Model file for the job. Use its own axes, mm. A direction names the side the tool comes from. Give positions to 0.01 mm unless a question says otherwise; leave off trailing zeros. Loops run counter-clockwise (first coordinate to the right, second up) from the corner with the lowest first, then second, coordinate; pieces in that order, holes last. Notation, with made-up numbers: (5, -39.75) -> (61, -39.75) arc R22 cw to (61, -19.75) -> close; hole circle Ø2 at (62.25, 73.25). An arc over 180 degrees is marked (long way). Use CSV: the item, a comma, the result in double quotes. Start each with the question number.
(1) Cut at C-C on y = 44. Write the cut outline in (x, z), then the cut area to 3 significant figures.
(2) Flat gauge pin, fed straight in: pin 1 (7.5 mm diameter, centred on x = 19.5, y = -65, fed in from +Z). Where does the tip first touch, or does it go through?
(3) Cut at A-A on y = -65. Write the cut outline in (x, z), then the cut area to 3 significant figures.
(4) 3-axis set-ups, long thin cutter, end or side, ignore diameter. For faces 4 (the flat face through (-21.4, -65.2, 3)), 5 (the flat face through (-19, 60, 1)), 6 (the flat face through (25.2, 0.3, 10)): which of +Z, -Z, +X, -X, +Y, -Y reach the whole face in a straight line?
(5) Drill centre lines: probe 1 along Y at (x, z) = (-19, 1.7); probe 2 along X at (y, z) = (65, 1.85); probe 3 along X at (y, z) = (-62.5, 3.75). Where is each one in solid material? Low to high.
(6) Cut at B-B on x = 4. Write the cut outline in (y, z).
(7) Cut at D-D on z = 6.25. Write the cut outline in (x, y), then the cut area to 3 significant figures.
(8) Pull direction X, two halves, no side cores. Call faces 1 (the flat face through (0, 70, 5)), 2 (the flat face through (26, 6, 0)), 3 (the flat face through (-27, -1, 4)): pulls with the +X half, pulls with the -X half, needs draft (parallel to the pull), parting line crosses it, or undercut.
Solid Edge part; units mm, degrees
sketch "Sketch1" plane through (0, 0, 0) normal (0, 0, 1) x (1, 0, 0)
  line L0 (27, -73) -> (-27, -73)
  line L1 (-27, -73) -> (-27, 73)
  line L2 (-27, 73) -> (27, 73)
  line L3 (27, 73) -> (27, -73)
  dimension "D1" = 27
  dimension "D2" = 27
extrude "Protrusion1" add sketch "Sketch1" along normal blind 10
sketch "Sketch2" plane through (0, 0, 10) normal (0, 0, 1) x (1, 0, 0)
  line L0 (24, -70) -> (-24, -70)
  line L1 (-24, -70) -> (-24, 70)
  line L2 (-24, 70) -> (24, 70)
  line L3 (24, 70) -> (24, -70)
  dimension "D1" = 24
  dimension "D2" = 24
extrude "Extrusionsausschnitt_1" cut sketch "Sketch2" along normal mid plane 76
fillet "Verrundung_1" radius 1 12 edges at (0, -73, 10) (-24, 0, 10) (-27, 0, 10) (0, -70, 10) (24, 0, 10) (27, 0, 10) (0, 73, 10) (0, 70, 10) (-27, 73, 5) (27, 73, 5) (27, -73, 5) (-27, -73, 5)
sketch "Sketch3" plane through (0, 0, 0) normal (0, 0, 1) x (1, 0, 0)
  line L0 (-14, -70) -> (-14, -60)
  line L1 (-14, -60) -> (-24, -60)
  line L2 (-24, -70) -> (-24, -60)
  line L3 (-14, -70) -> (-24, -70)
  dimension "D1" = 14
  dimension "D2" = 14
extrude "Extrusionsausprägung_2" add sketch "Sketch3" along normal blind 3
mirror "Mirror1" about plane through (0, 0, 0) normal (0, -1, 0) of "Extrusionsausprägung_2"
mirror "Mirror2" about plane through (0, 0, 0) normal (1, 0, 0) of "Mirror1", "Extrusionsausprägung_2"
hole "Bohrung_1" at (-19, -65, 3) direction (0, 0, -1) diameter 4.134 end through all
hole "Hole1" at (19, -65, 3) direction (0, 0, -1) diameter 4.134 end through all
hole "Hole2" at (19, 65, 3) direction (0, 0, -1) diameter 4.134 end through all
hole "Hole3" at (-19, 65, 3) direction (0, 0, -1) diameter 4.134 end through all
fillet "Verrundung_2" radius 0.5 8 edges at (-19, -60, 3) (-14, -65, 3) (14, -65, 3) (19, -60, 3) (-19, 60, 3) (-14, 65, 3) (14, 65, 3) (19, 60, 3)
properties part number "041" material "PLA"
Check result:
1,outline,"(-27, 0) -> (-24, 0) -> (-24, 9) arc R1 ccw to (-25, 10) -> (-26, 10) arc R1 ccw to (-27, 9) -> close; (24, 0) -> (27, 0) -> (27, 9) arc R1 ccw to (26, 10) -> (25, 10) arc R1 ccw to (24, 9) -> close"
1,area,"59.1 mm²"
2,pin 1,"z = 3"
3,outline,"(-27, 0) -> (-21.07, 0) -> (-21.07, 3) -> (-24, 3) -> (-24, 9) arc R1 ccw to (-25, 10) -> (-26, 10) arc R1 ccw to (-27, 9) -> close; (-16.93, 0) -> (-14, 0) -> (-14, 2.5) arc R0.5 ccw to (-14.5, 3) -> (-16.93, 3) -> close; (14, 0) -> (16.93, 0) -> (16.93, 3) -> (14.5, 3) arc R0.5 ccw to (14, 2.5) -> close; (21.07, 0) -> (27, 0) -> (27, 9) arc R1 ccw to (26, 10) -> (25, 10) arc R1 ccw to (24, 9) -> (24, 3) -> (21.07, 3) -> close"
3,area,"94.2 mm²"
4,face 4,"+Z"
4,face 5,"+Z, -Z"
4,face 6,"+Z, +X, -X, +Y, -Y"
5,probe 1,"-73 to -67.07, -62.93 to -60, 60 to 62.93, 67.07 to 73"
5,probe 2,"-27 to -21.07, -16.93 to -14, 14 to 16.93, 21.07 to 27"
5,probe 3,"-27 to -24, 24 to 27"
6,outline,"(-73, 0) -> (-70, 0) -> (-70, 9) arc R1 ccw to (-71, 10) -> (-72, 10) arc R1 ccw to (-73, 9) -> close; (70, 0) -> (73, 0) -> (73, 9) arc R1 ccw to (72, 10) -> (71, 10) arc R1 ccw to (70, 9) -> close"
7,outline,"(-27, -72) arc R1 ccw to (-26, -73) -> (26, -73) arc R1 ccw to (27, -72) -> (27, 72) arc R1 ccw to (26, 73) -> (-26, 73) arc R1 ccw to (-27, 72) -> close; hole (-24, -70) -> (24, -70) -> (24, 70) -> (-24, 70) -> close"
7,area,"1,160 mm²"
8,face 1,"undercut"
8,face 2,"needs draft"
8,face 3,"pulls with the -X half"
